```python
from build123d import *

# Parameters (mm, degrees)
SKETCH1_W             = 23
SKETCH1_H             = 21
EXTRUDE1_DEPTH        = 5
SKETCH2_R             = 2.15
EXTRUDE2_DEPTH        = 4.5
SKETCH4_R             = 1.25
EXTRUDE4_DEPTH        = 8
FILLET1_R             = 5
SKETCH6_R             = 4.5
EXTRUDE6_DEPTH        = 4.5
SKETCH9_W             = 12
SKETCH9_H             = 26
EXTRUDE9_DEPTH        = 5
SKETCH10_R            = 2
EXTRUDE10_DEPTH       = 4
SKETCH11_R            = 1.5
EXTRUDE11_DEPTH       = 5
M3_TAPPED_HOLE1_D     = 2.5
M3_TAPPED_HOLE1_DEPTH = 8
M3_TAPPED_HOLE1_TIP   = 0.751075774
EXTRUDE12_DEPTH       = 4
FILLET3_R             = 3
EXTRUDE14_DEPTH       = 4
FILLET4_R             = 2
EXTRUDE15_DEPTH       = 5
FILLET6_R             = 2


with BuildPart() as part:
    # Sketch1 → Extrude1 (new body)
    with BuildSketch(Plane.XY):
        with Locations((3.5, -4)):
            Rectangle(SKETCH1_W, SKETCH1_H)
    extrude(amount=EXTRUDE1_DEPTH)

    # Sketch2 → Extrude2 (cut)
    with BuildSketch(Plane.XY.offset(5)):
        Circle(SKETCH2_R)
    extrude(amount=-EXTRUDE2_DEPTH, mode=Mode.SUBTRACT)

    # Sketch4 → Extrude4 (cut)
    with BuildSketch(Plane.XZ.offset(14.5)):
        with Locations(Location((-1.4, 2.5, 0), (0, 0, 270))):
            Circle(SKETCH4_R)
        with Locations(Location((12, 2.5, 0), (0, 0, 270))):
            Circle(SKETCH4_R)
    extrude(amount=-EXTRUDE4_DEPTH, mode=Mode.SUBTRACT)

    # Fillet1
    fillet1_edges = [part.edges().sort_by_distance(p)[0] for p in [
        (15, 6.5, 2.5),
    ]]
    fillet(fillet1_edges, radius=FILLET1_R)

    # Sketch6 → Extrude6 (cut)
    with BuildSketch(Plane(origin=(0, 0, 0), x_dir=(-1, 0, 0), z_dir=(0, 0, -1))):
        with Locations((-4.9, -6.5)):
            Circle(SKETCH6_R)
    extrude(amount=-EXTRUDE6_DEPTH, mode=Mode.SUBTRACT)

    # Sketch9 → Extrude9 (add)
    with BuildSketch(Plane(origin=(0, 0, 0), x_dir=(-1, 0, 0), z_dir=(0, 0, -1))):
        with Locations((14, -6.5)):
            Rectangle(SKETCH9_W, SKETCH9_H)
    extrude(amount=-EXTRUDE9_DEPTH)

    # Sketch10 → Extrude10 (cut)
    with BuildSketch(Plane.XY.offset(5)):
        with Locations((-17, 1.5)):
            Circle(SKETCH10_R)
    extrude(amount=-EXTRUDE10_DEPTH, mode=Mode.SUBTRACT)

    # Sketch11 → Extrude11 (cut)
    with BuildSketch(Plane.XY.offset(5)):
        with Locations((-17.5, -5.5)):
            Circle(SKETCH11_R)
    extrude(amount=-EXTRUDE11_DEPTH, mode=Mode.SUBTRACT)

    # M3 Tapped Hole1
    with Locations(Plane(origin=(-1.4, -14.5, 2.5), x_dir=(0, 0, -1), z_dir=(0, -1, 0))):
        with Locations((0, 0), (0, 13.4)):
            Hole(M3_TAPPED_HOLE1_D / 2, depth=M3_TAPPED_HOLE1_DEPTH)
            with Locations((0, 0, -(M3_TAPPED_HOLE1_DEPTH + M3_TAPPED_HOLE1_TIP / 2))):  # 118° drill point
                Cone(0, M3_TAPPED_HOLE1_D / 2, M3_TAPPED_HOLE1_TIP, mode=Mode.SUBTRACT)

    # Sketch13 → Extrude12 (add)
    with BuildSketch(Plane(origin=(0, 0, 0), x_dir=(-1, 0, 0), z_dir=(0, 0, -1))):
        Polygon((20, -19.5), (8, -19.5), (8, -14.5), (2, -14.5), (2, -11.07), (18.1, 1), (20, 1), align=None)
    extrude(amount=EXTRUDE12_DEPTH)

    # Fillet3
    fillet3_edges = [part.edges().sort_by_distance(p)[0] for p in [
        (-20, -19.5, 0.5),
        (-20, 6.5, 2.5),
    ]]
    fillet(fillet3_edges, radius=FILLET3_R)

    # Sketch14 → Extrude14 (cut)
    with BuildSketch(Plane(origin=(0, 0, -4), x_dir=(-1, 0, 0), z_dir=(0, 0, -1))):
        Polygon((19.5, 1), (19.5, -7.5), (15.5, -7.5), (15.5, -0.949192547), (18.1, 1), align=None)
    extrude(amount=-EXTRUDE14_DEPTH, mode=Mode.SUBTRACT)

    # Fillet4
    fillet4_edges = [part.edges().sort_by_distance(p)[0] for p in [
        (-19.5, -7.5, -2),
        (-15.5, -7.5, -2),
    ]]
    fillet(fillet4_edges, radius=FILLET4_R - 0.0001)  # a hair under: the kernel refuses the full size

    # Sketch15 → Extrude15 (cut)
    with BuildSketch(Plane.XY.offset(5)):
        Polygon((-14, 2.5), (-17, 6.5), (-7, 6.5), (-10, 2.5), align=None)
    extrude(amount=-EXTRUDE15_DEPTH, mode=Mode.SUBTRACT)

    # Fillet6
    fillet6_edges = [part.edges().sort_by_distance(p)[0] for p in [
        (-10, 2.5, 2.5),
        (-14, 2.5, 2.5),
    ]]
    fillet(fillet6_edges, radius=FILLET6_R)


solid = part.part
```
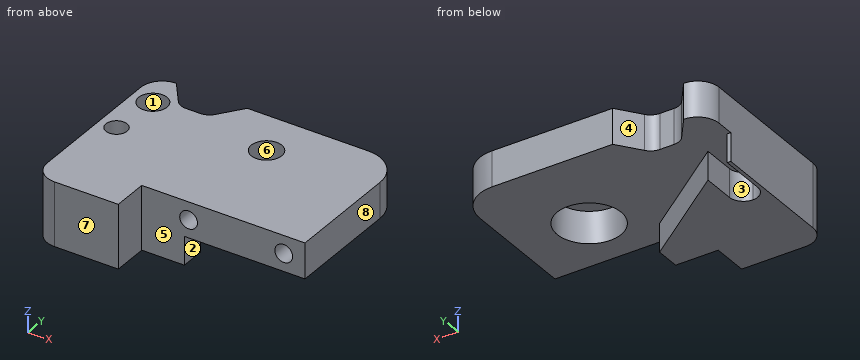
For this review, take the finished solid that the model builds, in its own axes (mm). Face numbers are marked on the shaded views. A direction names the side the tool comes from. Coordinates: 2 decimals unless noted, no trailing zeros. Write each loop counter-clockwise with the first axis right and the second up, starting at its lowest first coordinate (ties: lowest second). Pieces come first, ordered by that corner, then holes. Notation, with made-up numbers: (-7.5, 36.5) - (27.5, 36.5) arc R20 ccw to (27.5, 44.5) - close; hole circle Ø10 at (38.25, 53). An arc over 180 degrees is marked (long way). Answer in a Markdown table with one row per item. Add a question column.
Q1. For probe 1 along X at (y, z) = (-11.25, 2.5); probe 2 along Y at (x, z) = (4.9, 2.8); probe 3 along X at (y, z) = (1.75, 2.75), list the stretches that pass through material, from the lowest coordinate up.
Q2. We need section B-B, the plane x = 4.9. State the section outline as (y, z) points.
Q3. Tool access review of the marked faces 1, 2, 3, 4 and 5: name each direction out of +Z, -Z, +X, -X, +Y, -Y from which nothing blocks a thin tool from reaching the whole face with its end or side.
Q4. We need section A-A, the plane y = -5. State the section outline as (x, z) points.
Q5. We need section D-D, the plane y = -8.25. State the section outline as (x, z) points, and give its area (3 significant figures).
Q6. Draft analysis for pull direction Y (two halves, no side actions). For the marked faces 6, 7 and 8, state which applies: +Y half, -Y half, draft (parallel to the pull), parting line (faces both ways), or undercut.
Q7. For P1, Ø0.6, axis at x = -19.5, z = -1.5, coming from the +Y side; P2, Ø4.5, axis at y = -1.5, z = -2.5, coming from the +X side; P3, Ø8, axis at x = 9.5, y = -5, coming from the -Z side, all flat-tipped, find the tip position at first contact; note any pin that passes through.
Answer list:
| question | item | result |
|---|---|---|
| 1 | probe 1 | x = -20 to -2.65, -0.15 to 10.75, 13.25 to 15 |
| 1 | probe 2 | y = -14.5 to -11, -2 to 6.5 |
| 1 | probe 3 | x = -20 to -18.98, -15.02 to -1.25, 1.25 to 14.99 |
| 2 | outline | (-14.5, 0) - (-11, 0) - (-11, 4.5) - (-2, 4.5) - (-2, 0) - (6.5, 0) - (6.5, 5) - (-14.5, 5) - close |
| 3 | face 1 | +Z |
| 3 | face 2 | -Z, +X, +Y, -Y |
| 3 | face 3 | -Z, +Y |
| 3 | face 4 | +Z, -Z, +Y |
| 3 | face 5 | +Z, -Z, +X, -Y |
| 4 | outline | (-20, -4) - (-19.5, -4) - (-19.5, 0) - (-18.91, 0) - (-18.91, 5) - (-20, 5) - close; (-16.09, 0) - (-15.5, 0) - (-15.5, -4) - (-10.1, -4) - (-10.1, 0) - (0.66, 0) - (0.66, 4.5) - (9.14, 4.5) - (9.14, 0) - (15, 0) - (15, 5) - (-16.09, 5) - close |
| 5 | outline | (-20, -4) - (-5.76, -4) - (-5.76, 0) - (0.75, 0) - (0.75, 4.5) - (9.05, 4.5) - (9.05, 0) - (15, 0) - (15, 5) - (-20, 5) - close; hole circle Ø2.5 at (-1.4, 2.5); hole circle Ø2.5 at (12, 2.5) |
| 5 | area | 185 mm2 |
| 6 | face 6 | undercut |
| 6 | face 7 | -Y half |
| 6 | face 8 | draft |
| 7 | P1 | stops at y = 1 |
| 7 | P2 | stops at x = -11.76 |
| 7 | P3 | stops at z = 0 |
